from build123d import *

# Parameters (mm, degrees)
SKETCH2_R           = 21.5
BOSS_EXTRUDE1_DEPTH = 3
CUT_EXTRUDE1_DEPTH  = 4.0000001
SKETCH4_R           = 1.6
CUT_EXTRUDE2_DEPTH  = 4.0000001
CUT_EXTRUDE3_DEPTH  = 4.0000001
BOSS_EXTRUDE3_DEPTH = 3
FILLET1_R           = 3
SKETCH7_R           = 4
CUT_EXTRUDE4_DEPTH  = 4.0000001


with BuildPart() as part:
    # Sketch2 → Boss-Extrude1 (new body)
    with BuildSketch(Plane.ZY.offset(80.1)):
        with BuildLine():
            ThreePointArc((-17.093145751, 29.75), (-18.62387948, 29.44551813), (-19.921572875, 28.578427125))
            Line((-19.921572875, 28.578427125), (-22.578427125, 25.921572875))
            ThreePointArc((-22.578427125, 25.921572875), (-23.44551813, 24.62387948), (-23.75, 23.093145751))
            Line((-23.75, 23.093145751), (-23.75, 19.635890143))
            ThreePointArc((-23.75, 19.635890143), (-23.958769179, 15.071535497), (-24.583333333, 10.545296714))
            ThreePointArc((-24.583333333, 10.545296714), (-24.89561541, 8.282177323), (-25, 6))
            Line((-25, 6), (-25, -18.013516259))
            add(Edge.make_bspline(
                [(-25, -18.013516259), (-25, -19.75), (-24.760179539, -21.458720786)],
                knots=[4.71238898, 4.71238898, 4.71238898, 4.891446603, 4.891446603, 4.891446603], degree=2, weights=[1, 0.995994972, 1]))
            Line((-24.760179539, -21.458720786), (-23.936908844, -27.324524486))
            add(Edge.make_bspline(
                [(-23.936908844, -27.324524486), (-20.894736842, -49), (-8.26270655, -49)],
                knots=[1.708421538, 1.708421538, 1.708421538, 3.107039678, 3.107039678, 3.107039678], degree=2, weights=[1, 0.765287114, 1]))
            Line((-8.26270655, -49), (8.26270655, -49))
            add(Edge.make_bspline(
                [(8.26270655, -49), (20.894736842, -49), (23.936908844, -27.324524486)],
                knots=[0.034552975, 0.034552975, 0.034552975, 1.433171116, 1.433171116, 1.433171116], degree=2, weights=[1, 0.765287114, 1]))
            Line((23.936908844, -27.324524486), (24.760179539, -21.458720786))
            add(Edge.make_bspline(
                [(24.760179539, -21.458720786), (25, -19.75), (25, -18.013516259)],
                knots=[1.391738704, 1.391738704, 1.391738704, 1.570796327, 1.570796327, 1.570796327], degree=2, weights=[1, 0.995994972, 1]))
            Line((25, -18.013516259), (25, 6))
            ThreePointArc((25, 6), (24.89561541, 8.282177323), (24.583333333, 10.545296714))
            ThreePointArc((24.583333333, 10.545296714), (23.958769179, 15.071535497), (23.75, 19.635890143))
            Line((23.75, 19.635890143), (23.75, 23.093145751))
            ThreePointArc((23.75, 23.093145751), (23.44551813, 24.62387948), (22.578427125, 25.921572875))
            Line((22.578427125, 25.921572875), (19.921572875, 28.578427125))
            ThreePointArc((19.921572875, 28.578427125), (18.62387948, 29.44551813), (17.093145751, 29.75))
            Line((17.093145751, 29.75), (-17.093145751, 29.75))
        make_face()
        with Locations((0, 6)):
            Circle(SKETCH2_R, mode=Mode.SUBTRACT)
    extrude(amount=BOSS_EXTRUDE1_DEPTH)

    # Sketch3 → Cut-Extrude1 (cut, through all)
    with BuildSketch(Plane.ZY.offset(83.1)):
        with BuildLine():
            ThreePointArc((-15.196569313, 25.146541488), (-15.032451192, 26.906673654), (-16.792583358, 27.070791775))
            ThreePointArc((-16.792583358, 27.070791775), (-18.571456346, 25.459260737), (-20.203027197, 23.698750028))
            ThreePointArc((-20.203027197, 23.698750028), (-20.058850519, 21.936872312), (-18.296972803, 22.081048991))
            ThreePointArc((-18.296972803, 22.081048991), (-16.813726575, 23.681513271), (-15.196569313, 25.146541488))
        make_face()
        with BuildLine():
            ThreePointArc((-19.691847489, -13.623229665), (-19.657568517, -13.657568517), (-19.623229665, -13.691847489))
            ThreePointArc((-19.623229665, -13.691847489), (-17.643333693, -13.688391915), (-17.646789267, -11.708495943))
            ThreePointArc((-17.646789267, -11.708495943), (-17.67766953, -11.67766953), (-17.708495943, -11.646789267))
            ThreePointArc((-17.708495943, -11.646789267), (-19.688391915, -11.643333693), (-19.691847489, -13.623229665))
        make_face()
        with BuildLine():
            ThreePointArc((17.646789267, -11.708495943), (17.67766953, -11.67766953), (17.708495943, -11.646789267))
            ThreePointArc((17.708495943, -11.646789267), (19.688391915, -11.643333693), (19.691847489, -13.623229665))
            ThreePointArc((19.691847489, -13.623229665), (19.657568517, -13.657568517), (19.623229665, -13.691847489))
            ThreePointArc((19.623229665, -13.691847489), (17.643333693, -13.688391915), (17.646789267, -11.708495943))
        make_face()
        with BuildLine():
            ThreePointArc((18.296972803, 22.081048991), (16.813726575, 23.681513271), (15.196569313, 25.146541488))
            ThreePointArc((15.196569313, 25.146541488), (15.032451192, 26.906673654), (16.792583358, 27.070791775))
            ThreePointArc((16.792583358, 27.070791775), (18.571456346, 25.459260737), (20.203027197, 23.698750028))
            ThreePointArc((20.203027197, 23.698750028), (20.058850519, 21.936872312), (18.296972803, 22.081048991))
        make_face()
    extrude(amount=-CUT_EXTRUDE1_DEPTH, mode=Mode.SUBTRACT)

    # Sketch4 → Cut-Extrude2 (cut, through all)
    with BuildSketch(Plane(origin=(-80.1, 0, 0), x_dir=(0, 0, -1), z_dir=(1, 0, 0))):
        with Locations((0, -35)):
            Circle(SKETCH4_R)
    extrude(amount=-CUT_EXTRUDE2_DEPTH, mode=Mode.SUBTRACT)

    # Sketch5 → Cut-Extrude3 (cut, through all)
    with BuildSketch(Plane(origin=(-80.1, 0, 0), x_dir=(0, 0, -1), z_dir=(1, 0, 0))):
        with BuildLine():
            Line((-19.521169673, -21.8125), (-5.284461571, -21.8125))
            ThreePointArc((-5.284461571, -21.8125), (-4.284461571, -22.8125), (-5.284461571, -23.8125))
            Line((-5.284461571, -23.8125), (-19.521169673, -23.8125))
            ThreePointArc((-19.521169673, -23.8125), (-20.521169673, -22.8125), (-19.521169673, -21.8125))
        make_face()
        with BuildLine():
            Line((-18.950227736, -25.875), (-7.838149252, -25.875))
            ThreePointArc((-7.838149252, -25.875), (-6.838149252, -26.875), (-7.838149252, -27.875))
            Line((-7.838149252, -27.875), (-18.950227736, -27.875))
            ThreePointArc((-18.950227736, -27.875), (-19.950227736, -26.875), (-18.950227736, -25.875))
        make_face()
        with BuildLine():
            Line((-16.793141988, -34), (-6, -34))
            ThreePointArc((-6, -34), (-5, -35), (-6, -36))
            Line((-6, -36), (-16.793141988, -36))
            ThreePointArc((-16.793141988, -36), (-17.793141988, -35), (-16.793141988, -34))
        make_face()
        with BuildLine():
            Line((-10, -38.0625), (10, -38.0625))
            ThreePointArc((10, -38.0625), (11, -39.0625), (10, -40.0625))
            Line((10, -40.0625), (-10, -40.0625))
            ThreePointArc((-10, -40.0625), (-11, -39.0625), (-10, -38.0625))
        make_face()
        with BuildLine():
            Line((-18.129953736, -29.9375), (-5.690263266, -29.9375))
            ThreePointArc((-5.690263266, -29.9375), (-4.690263266, -30.9375), (-5.690263266, -31.9375))
            Line((-5.690263266, -31.9375), (-18.129953736, -31.9375))
            ThreePointArc((-18.129953736, -31.9375), (-19.129953736, -30.9375), (-18.129953736, -29.9375))
        make_face()
        with BuildLine():
            Line((19.521169673, -21.8125), (5.284461571, -21.8125))
            ThreePointArc((5.284461571, -21.8125), (4.284461571, -22.8125), (5.284461571, -23.8125))
            Line((5.284461571, -23.8125), (19.521169673, -23.8125))
            ThreePointArc((19.521169673, -23.8125), (20.521169673, -22.8125), (19.521169673, -21.8125))
        make_face()
        with BuildLine():
            Line((18.950227736, -25.875), (7.838149252, -25.875))
            ThreePointArc((7.838149252, -25.875), (6.838149252, -26.875), (7.838149252, -27.875))
            Line((7.838149252, -27.875), (18.950227736, -27.875))
            ThreePointArc((18.950227736, -27.875), (19.950227736, -26.875), (18.950227736, -25.875))
        make_face()
        with BuildLine():
            Line((16.793141988, -34), (6, -34))
            ThreePointArc((6, -34), (5, -35), (6, -36))
            Line((6, -36), (16.793141988, -36))
            ThreePointArc((16.793141988, -36), (17.793141988, -35), (16.793141988, -34))
        make_face()
        with BuildLine():
            Line((18.129953736, -29.9375), (5.690263266, -29.9375))
            ThreePointArc((5.690263266, -29.9375), (4.690263266, -30.9375), (5.690263266, -31.9375))
            Line((5.690263266, -31.9375), (18.129953736, -31.9375))
            ThreePointArc((18.129953736, -31.9375), (19.129953736, -30.9375), (18.129953736, -29.9375))
        make_face()
    extrude(amount=-CUT_EXTRUDE3_DEPTH, mode=Mode.SUBTRACT)

    # Sketch6 → Boss-Extrude3 (add)
    with BuildSketch(Plane.ZY.offset(83.1)):
        with BuildLine():
            Line((-21.5, 2), (-10.514870422, 2))
            ThreePointArc((-10.514870422, 2), (-11.25, 6), (-10.514870422, 10))
            Line((-10.514870422, 10), (-21.5, 10))
            Line((-21.5, 10), (-21.5, 2))
        make_face()
        with BuildLine():
            Line((-10.514870422, 2), (10.514870422, 2))
            ThreePointArc((10.514870422, 2), (11.064691416, 3.966504518), (11.25, 6))
            ThreePointArc((11.25, 6), (11.064691416, 8.033495482), (10.514870422, 10))
            Line((10.514870422, 10), (-10.514870422, 10))
            ThreePointArc((-10.514870422, 10), (-11.25, 6), (-10.514870422, 2))
        make_face()
        with BuildLine():
            ThreePointArc((7.061208501, 3.284351593), (5.300168435, 3.438422635), (5.454239477, 5.199462701))
            ThreePointArc((5.454239477, 5.199462701), (7.215279543, 5.045391659), (7.061208501, 3.284351593))
        make_face(mode=Mode.SUBTRACT)
        with BuildLine():
            ThreePointArc((-5.454239477, 6.800537299), (-7.215279543, 6.954608341), (-7.061208501, 8.715648407))
            ThreePointArc((-7.061208501, 8.715648407), (-5.300168435, 8.561577365), (-5.454239477, 6.800537299))
        make_face(mode=Mode.SUBTRACT)
        with BuildLine():
            Line((-10.514870422, 10), (10.514870422, 10))
            ThreePointArc((10.514870422, 10), (0, 17.25), (-10.514870422, 10))
        make_face()
        with BuildLine():
            ThreePointArc((-10.514870422, 2), (0, -5.25), (10.514870422, 2))
            Line((10.514870422, 2), (-10.514870422, 2))
        make_face()
        with BuildLine():
            Line((10.514870422, 2), (21.5, 2))
            Line((21.5, 2), (21.5, 10))
            Line((21.5, 10), (10.514870422, 10))
            ThreePointArc((10.514870422, 10), (11.064691416, 8.033495482), (11.25, 6))
            ThreePointArc((11.25, 6), (11.064691416, 3.966504518), (10.514870422, 2))
        make_face()
    extrude(amount=-BOSS_EXTRUDE3_DEPTH)

    # Fillet1
    fillet1_edges = [part.edges().sort_by_distance(p)[0] for p in [
        (-81.6, 2, -21.124630174),
        (-81.6, 10, -21.124630174),
        (-81.6, 10, 21.124630174),
        (-81.6, 2, 21.124630174),
        (-81.6, 2, 10.514870422),
        (-81.6, 10, 10.514870422),
        (-81.6, 10, -10.514870422),
        (-81.6, 2, -10.514870422),
    ]]
    fillet(fillet1_edges, radius=FILLET1_R)

    # Sketch7 → Cut-Extrude4 (cut, through all)
    with BuildSketch(Plane(origin=(-80.1, 0, 0), x_dir=(0, 0, -1), z_dir=(1, 0, 0))):
        with Locations((0, 6)):
            Circle(SKETCH7_R)
    extrude(amount=-CUT_EXTRUDE4_DEPTH, mode=Mode.SUBTRACT)


solid = part.part
Can you work these out from the model? Positions are in its coordinate system, mm. Round coordinates to 2 decimals unless told otherwise and drop trailing zeros. Write each loop counter-clockwise with the first axis right and the second up, starting at its lowest first coordinate (ties: lowest second). Pieces come first, ordered by that corner, then holes. Notation, with made-up numbers: M 89.5,65 L 95.5,65 A22 cw 95.5,100 Z; hole C -5,48 d2. An arc over 180 degrees is marked long. Use a Markdown table: item, result.
Item 1: We'd pull the mould along Z, two halves only. Please class faces 1 (the face through (-81.579, -24.433, 24.343)), 2 (the face through (-82, -29.938, -12)): released by +Z, released by -Z, zero draft, split by the parting line, or undercut.
Found:
| item | result |
|---|---|
| face 1 | released by +Z |
| face 2 | undercut |
Item 2: I want a section at B-B (x = -81.05). State how many separate pieces and enclosed holes the cut face has, and give its area (3 significant figures).
Found:
| item | result |
|---|---|
| separate pieces | 1 |
| enclosed holes | 19 |
| area | 2,390 mm2 |
Item 3: For pin 1 Ø1.5 at (x, z) = (-82, 15.5) entering from -Y; pin 2 Ø1 at (x, z) = (-81.5, -18) entering from -Y; pin 3 Ø0.9 at (x, z) = (-81, -10.5) entering from -Y, each with a flat end and sliding along its axis, tell me the tip position at first contact or that it passes through.
Found:
| item | result |
|---|---|
| pin 1 | stops at y = -46.52 |
| pin 2 | stops at y = -43.75 |
| pin 3 | stops at y = -48.82 |
Item 4: I want a section at A-A (z = 0). List the corners of the cut face in (x, y) for me, and give its area (3 significant figures).
Found:
| item | result |
|---|---|
| outline | M -83.1,-49 L -80.1,-49 L -80.1,-40.06 L -83.1,-40.06 Z; M -83.1,-38.06 L -80.1,-38.06 L -80.1,-36.6 L -83.1,-36.6 Z; M -83.1,-33.4 L -80.1,-33.4 L -80.1,-15.5 L -83.1,-15.5 Z; M -83.1,-5.25 L -80.1,-5.25 L -80.1,2 L -83.1,2 Z; M -83.1,10 L -80.1,10 L -80.1,17.25 L -83.1,17.25 Z; M -83.1,27.5 L -80.1,27.5 L -80.1,29.75 L -83.1,29.75 Z |
| area | 135 mm2 |
Item 5: If I drill on line 1 along Y through (x, z) = (-82, 0); line 2 along Z through (x, y) = (-81.25, -2.5); line 3 along Z through (x, y) = (-82.8, -22.5), over which ranges is the centre line in solid material (lowest first)? Write a range as [from, to].
Found:
| item | result |
|---|---|
| line 1 | y = [-49, -40.06], [-38.06, -36.6], [-33.4, -15.5], [-5.25, 2], [10, 17.25], [27.5, 29.75] |
| line 2 | z = [-25, -19.75], [-7.37, 7.37], [19.75, 25] |
| line 3 | z = [-24.61, -20.47], [-4.33, 4.33], [20.47, 24.61] |
